Geometry: see drawing. Coordinates: mm, zero at the bounding-box minimum. A direction names the side the tool comes from. Round coordinates to 2 decimals unless told otherwise and drop trailing zeros. Order: outer loops, then holes, each group sorted by start corner. A loop starts at its lowest first (then second) coordinate and runs counter-clockwise, first axis right, second up. Notation, with made-up numbers: (55.5, 20) - (89.5, 20) arc R12 ccw to (89.5, 25) - close; hole circle Ø9 at (16, 75.25). An arc over 180 degrees is marked (long way). Put each result on its own line as item: value. Start each with the question number.
1) Section B-B on y = 30.5. Output: boundary loops of the cut face in (x, z).
2) Contact query for flat-ended pins moving along their axis: P1, Ø5.5, axis at x = 24.5, z = 8.5, coming from the +Y side; P2, Ø9, axis at y = 39, z = 12, coming from the -X side; P3, Ø9, axis at x = 21.5, z = 11, coming from the -Y side. Output: stop coordinate, or through.
3) Mould query, pull axis X, two halves, no side actions, for the marked faces 4, 5, 6 and 7. Classes: +X half, -X half, draft (parallel to the pull), parting line (faces both ways), or undercut.
4) Line query: probe 1 along Y at (x, z) = (46, 2); probe 2 along X at (y, z) = (55.5, 11); probe 3 along Z at (x, y) = (13, 19.5). Output: solid intervals per line, ascending. Write a range as [from, to].
5) Section A-A on z = 6.5. Output: boundary loops of the cut face in (x, y), then the cut area to 3 significant figures.
6) Access query for the marked faces 1, 2 and 3. Directions: +Z, -Z, +X, -X, +Y, -Y. A direction counts if a zero-diameter tool reaches every point of the face in a straight line with its end or side. Return the directions, or none.
7) Section C-C on x = 9. Output: boundary loops of the cut face in (y, z), then the cut area to 3 significant figures.
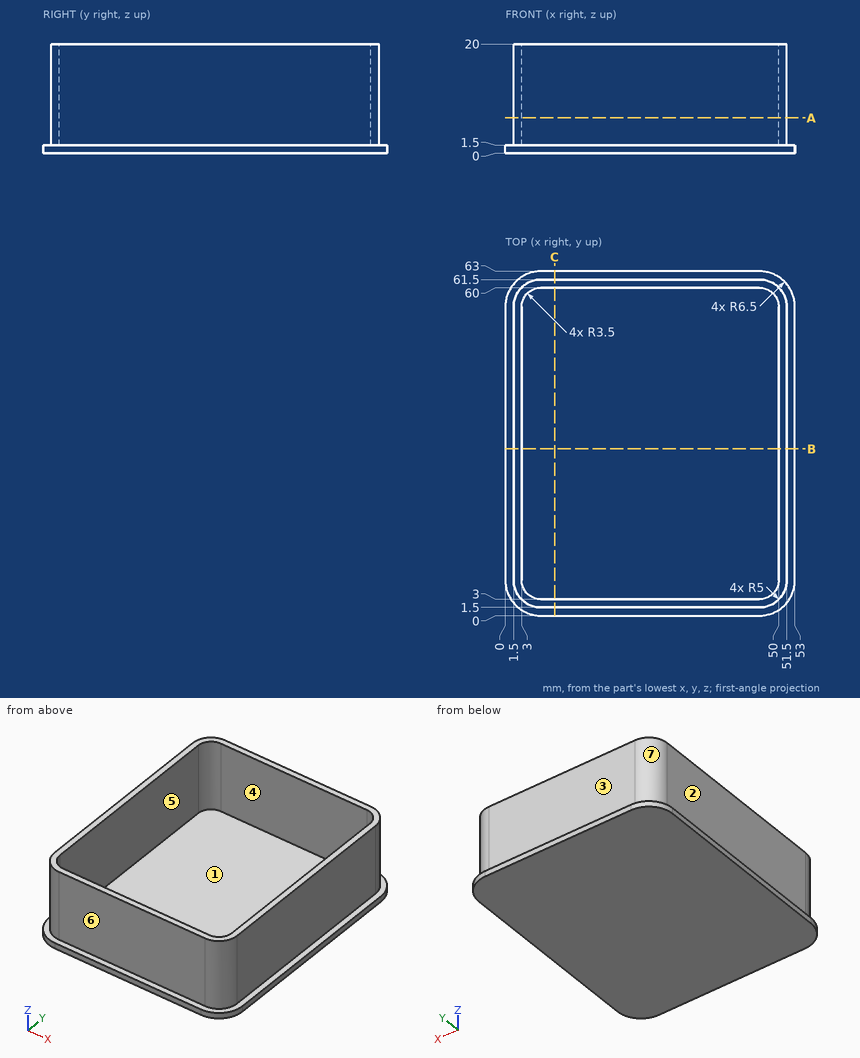
Answer sheet:
1. outline: (0, 0) - (53, 0) - (53, 1.5) - (51.5, 1.5) - (51.5, 20) - (50, 20) - (50, 1.5) - (3, 1.5) - (3, 20) - (1.5, 20) - (1.5, 1.5) - (0, 1.5) - close
2. P1: y = 61.5
2. P2: x = 1.5
2. P3: y = 1.5
3. face 4: undercut
3. face 5: undercut
3. face 6: draft
3. face 7: -X half
4. probe 1: [1.5, 3], [60, 61.5]
4. probe 2: [1.5, 3], [50, 51.5]
4. probe 3: [0, 1.5]
5. outline: (1.5, 6.5) arc R5 ccw to (6.5, 1.5) - (46.5, 1.5) arc R5 ccw to (51.5, 6.5) - (51.5, 56.5) arc R5 ccw to (46.5, 61.5) - (6.5, 61.5) arc R5 ccw to (1.5, 56.5) - close; hole (3, 6.5) arc R3.5 ccw to (6.5, 3) - (46.5, 3) arc R3.5 ccw to (50, 6.5) - (50, 56.5) arc R3.5 ccw to (46.5, 60) - (6.5, 60) arc R3.5 ccw to (3, 56.5) - close
5. area: 310 mm^2
6. face 1: +Z
6. face 2: +Z, -X, +Y, -Y
6. face 3: +Z, +X, -X, +Y
7. outline: (0, 0) - (63, 0) - (63, 1.5) - (61.5, 1.5) - (61.5, 20) - (60, 20) - (60, 1.5) - (3, 1.5) - (3, 20) - (1.5, 20) - (1.5, 1.5) - (0, 1.5) - close
7. area: 150 mm^2
